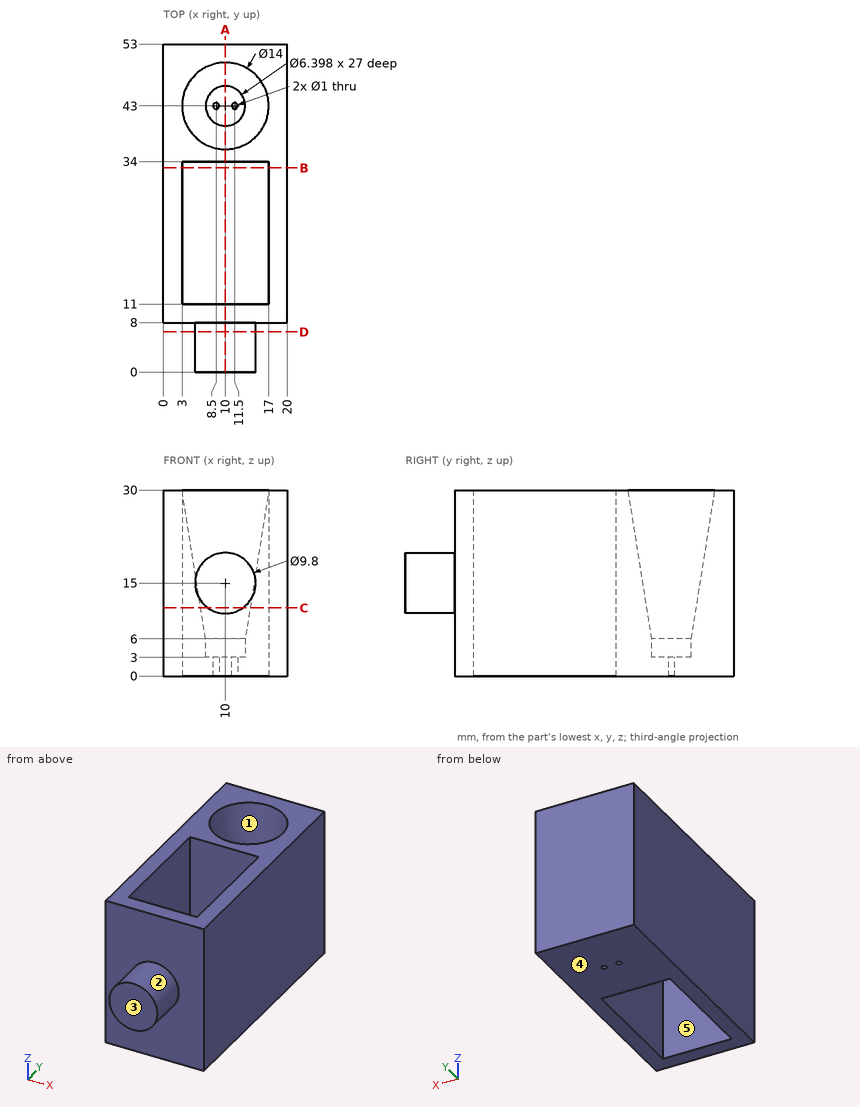
Check sheet for the drawn part. Datum: minimum x, y, z corner. Units: mm. A direction names the side the tool comes from. Give positions to 0.01 mm unless a question says otherwise; leave off trailing zeros. Order: outer loops, then holes, each group sorted by start corner. A loop starts at its lowest first (then second) coordinate and runs counter-clockwise, first axis right, second up. Notation, with made-up numbers: (22.25, -8) -> (38.25, -8) arc R12 cw to (38.25, 14) -> close; hole circle Ø7 at (-2, 11.25). An arc over 180 degrees is marked (long way). Use a Markdown table: item, result.
1) Section check D-D, the plane y = 6.5. Record the boundary of the cut face in (x, z).
Results:
| item | result |
|---|---|
| outline | circle Ø9.8 at (10, 15) |
2) Mould release check, pull along Y, two halves, no side actions. Record for the marked faces 1, 2 and 3: pulls with the +Y half, pulls with the -Y half, needs draft (parallel to the pull), parting line crosses it, or undercut.
Results:
| item | result |
|---|---|
| face 1 | undercut |
| face 2 | needs draft |
| face 3 | pulls with the -Y half |
3) Depth check by flat-ended pin: pin 1 Ø1 at (x, z) = (16, 26) entering from -Y; pin 2 Ø5 at (x, y) = (10, 43) entering from +Z. Enter the tip coordinate at first touch or a pass-through.
Results:
| item | result |
|---|---|
| pin 1 | y = 8 |
| pin 2 | z = 3 |
4) Section check B-B, the plane y = 33. Record the boundary of the cut face in (x, z).
Results:
| item | result |
|---|---|
| outline | (0, 0) -> (3, 0) -> (3, 30) -> (0, 30) -> close; (17, 0) -> (20, 0) -> (20, 30) -> (17, 30) -> close |
5) Section check C-C, the plane z = 11. Record the boundary of the cut face in (x, y), then the cut area to 3 significant figures.
Results:
| item | result |
|---|---|
| outline | (0, 8) -> (7.17, 8) -> (7.17, 0) -> (12.83, 0) -> (12.83, 8) -> (20, 8) -> (20, 53) -> (0, 53) -> close; hole (3, 11) -> (17, 11) -> (17, 34) -> (3, 34) -> close; hole circle Ø7.98 at (10, 43) |
| area | 573 mm² |
6) Section check A-A, the plane x = 10. Record the boundary of the cut face in (y, z).
Results:
| item | result |
|---|---|
| outline | (0, 10.1) -> (8, 10.1) -> (8, 0) -> (11, 0) -> (11, 30) -> (8, 30) -> (8, 19.9) -> (0, 19.9) -> close; (34, 0) -> (53, 0) -> (53, 30) -> (50, 30) -> (46.2, 6) -> (46.2, 3) -> (39.8, 3) -> (39.8, 6) -> (36, 30) -> (34, 30) -> close |
7) Tool access check on the marked faces 4 and 5. Record the directions out of +Z, -Z, +X, -X, +Y, -Y that give a thin tool (end or side, any length) a straight path to the whole face; none if there is none.
Results:
| item | result |
|---|---|
| face 4 | -Z, +X, -X, +Y, -Y |
| face 5 | +Z, -Z |
8) Material ranges on probe 1 along Y at (x, z) = (8.5, 1); probe 2 along X at (y, z) = (43, 1.25); probe 3 along Y at (x, z) = (10, 5.05), recorded low to high.
Results:
| item | result |
|---|---|
| probe 1 | 8 to 11, 34 to 42.5, 43.5 to 53 |
| probe 2 | 0 to 8, 9 to 11, 12 to 20 |
| probe 3 | 8 to 11, 34 to 39.8, 46.2 to 53 |
